Read the model definition and answer for the solid it produces. Units are mm, in the model's axes. Face numbers are marked on the shaded views. Coordinates: 2 decimals unless noted, no trailing zeros. Loops run counter-clockwise (first coordinate to the right, second up) from the corner with the lowest first, then second, coordinate; pieces in that order, holes last.
Q1. Section C-C (z = 23) is taken. Give the vertices of the cut face in (x, y).
Q2. The mould has two halves that part along Y. Classify the marked faces 1, 2, 3 and 4: pulls with the +Y half, pulls with the -Y half, needs draft (parallel to the pull), parting line crosses it, or undercut.
Q3. Section A-A (x = 0) is taken. Give the vertices of the cut face in (y, z).
Q4. Straight lines are drawn through the part: line 1 (Y direction, x = -6, z = 22.5); line 2 (Y direction, x = -2, z = 9.25); line 3 (X direction, y = 5.5, z = 6.5). For each, find the intervals that lie inside material, in ascending order.
from build123d import *

# Parameters (mm, degrees)
F0_W     = 44.030744
F0_H     = 44.030744
F1_DEPTH = 25.4


with BuildPart() as f1:
    # F0 (on Top) → F1 (new body)
    with BuildSketch(Plane.XY):
        Rectangle(F0_W, F0_H)
    extrude(amount=F1_DEPTH)


with BuildPart() as f3:
    # F2 (on Front) → F3 (revolve)
    with BuildSketch(Plane.XZ):
        Polygon((19.131194, 30.48), (0, 30.48), (0, -7.62), align=None)
    revolve(axis=Axis((0, 0, 11.43), (0, 0, 1)))


with BuildPart() as f1_1:
    add(f1.part)

    # F4: cut F3
    add(f3.part, mode=Mode.SUBTRACT)


solid = f1_1.part
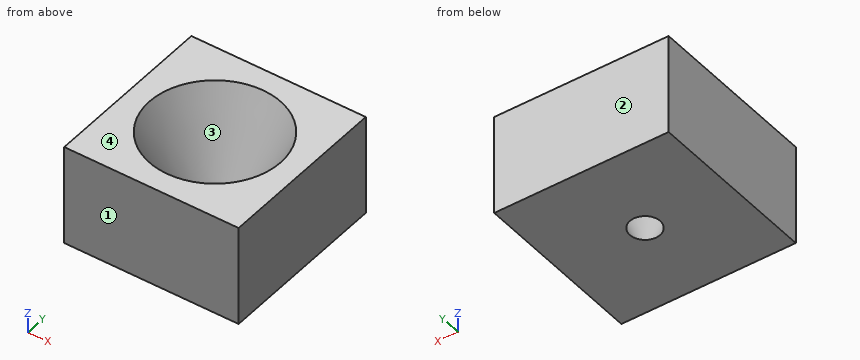
Numbers:
1. outline: (-22.02, -22.02) - (22.02, -22.02) - (22.02, 22.02) - (-22.02, 22.02) - close; hole circle Ø30.75 at (0, 0)
2. face 1: pulls with the -Y half
2. face 2: pulls with the +Y half
2. face 3: undercut
2. face 4: needs draft
3. outline: (-22.02, 0) - (-3.83, 0) - (-16.58, 25.4) - (-22.02, 25.4) - close; (3.83, 0) - (22.02, 0) - (22.02, 25.4) - (16.58, 25.4) - close
4. line 1: y = -22.02 to -13.88, 13.88 to 22.02
4. line 2: y = -22.02 to -8.23, 8.23 to 22.02
4. line 3: x = -22.02 to -4.47, 4.47 to 22.02
